Design review of the part built by this model. Coordinates are the model's own, in mm. A direction names the side the tool comes from. Coordinates: 2 decimals unless noted, no trailing zeros. Write each loop counter-clockwise with the first axis right and the second up, starting at its lowest first coordinate (ties: lowest second). Pieces come first, ordered by that corner, then holes. Notation, with made-up numbers: M -33,-36 L -25,-36 A34 cw -25,3 Z; hole C -31.5,-20.75 d11. An arc over 180 degrees is marked long. Write each question's results on one line, items separated by ' | '. Start each with the question number.
```python
from build123d import *

# Parameters (mm, degrees)
FILLET1_R       = 0.1
SKETCH3_W       = 0.74
SKETCH3_H       = 2.8
SKETCH4_W       = 0.74
SKETCH4_H       = 1.054964664
RECPAT_COUNT    = 2
RECPAT_ANGLE    = 90
THDSCHPAT_COUNT = 7
THDSCHPAT_PITCH = 0.5


with BuildPart() as part:
    # BodySke → Base-Revolve (revolve)
    with BuildSketch(Plane.XY):
        with BuildLine():
            Line((2.4, 1.5), (2.4, 2.8))
            Line((2.4, 2.8), (1.003501533, 2.8))
            ThreePointArc((1.003501533, 2.8), (0.873295971, 2.76653015), (0.775371599, 2.674418605))
            ThreePointArc((0.775371599, 2.674418605), (0.197753546, 1.392274756), (0, 0))
            Line((0, 0), (6.4, 0))
            Line((6.4, 0), (6.4, 1.5))
            Line((6.4, 1.5), (2.4, 1.5))
        make_face()
    revolve(axis=Axis((-25.4, 0, 0), (1, 0, 0)))

    # Fillet1
    fillet1_edges = [part.edges().sort_by_distance(p)[0] for p in [
        (2.4, -1.5, 0),
    ]]
    fillet(fillet1_edges, radius=FILLET1_R)

    # Sketch3 → Recess section 0
    with BuildSketch(Plane(origin=(0, 0, 0), x_dir=(0, 0, -1), z_dir=(1, 0, 0))):
        Rectangle(SKETCH3_W, SKETCH3_H)
    # Sketch4 → Recess section 1
    with BuildSketch(Plane(origin=(1.75, 0, 0), x_dir=(0, 0, -1), z_dir=(1, 0, 0))):
        Rectangle(SKETCH4_W, SKETCH4_H)
    recess = loft(mode=Mode.SUBTRACT)

    # RecPat: Recess ×2 about axis
    recpat_axis = Axis((0, 0, 0), (1, 0, 0))
    for i in range(1, RECPAT_COUNT):
        add(recess.rotate(recpat_axis, i * RECPAT_ANGLE / (RECPAT_COUNT - 1)), mode=Mode.SUBTRACT)

    # RecCorSke → RecessCore (revolve, cut)
    with BuildSketch(Plane.XY):
        Polygon((0, 0), (0, 0.678371921), (1.75, 0.556), (1.930655351, 0), align=None)
    revolve(axis=Axis((-3.175, 0, 0), (1, 0, 0)), mode=Mode.SUBTRACT)

    # ThdSchSke → ThreadSchematic (revolve, cut)
    with BuildSketch(Plane.XY):
        Polygon((3.4, -1.2195), (3.203591786, -1.5), (3.203591786, -1.875), (3.596408214, -1.875), (3.596408214, -1.5), align=None)
    threadschematic = revolve(axis=Axis((-3.175, 0, 0), (1, 0, 0)), mode=Mode.SUBTRACT)

    # ThdSchPat: ThreadSchematic ×7
    with Locations(*[(i * THDSCHPAT_PITCH, 0, 0) for i in range(1, THDSCHPAT_COUNT)]):
        add(threadschematic, mode=Mode.SUBTRACT)


solid = part.part
```
Item 1: For faces 1 (the conical face through (1.92, 0.03, 0.01)), 2 (the flat face through (2.4, 0, -2)), list the 3-axis set-ups (+Z, -Z, +X, -X, +Y, -Y) from which the entire face can be reached by the end or side of a thin tool; tool diameter is ignored.
Item 2: We need section A-A on z = 1.4. Count the separate pieces of the cut face and the enclosed holes in it, then the cut area to 3 significant figures.
Item 3: We need section B-B on x = 4.5. State the section outline as (y, z) points.
Item 4: Insertion check: pin 1 Ø1.5 at (x, y) = (5, -1) entering from -Z; pin 2 Ø3 at (y, z) = (-1.5, -1.5) entering from -X; pin 3 Ø3 at (x, z) = (3.5, 2) entering from +Y. Each pin has a flat end and moves straight along its axis. Give the tip position at first contact, or say it passes through.
Item 5: Wall thickness on L1, parallel to X at y = -0.7, z = -1.75; L2, parallel to Z at x = 0.5, y = -1.05; L3, parallel to Z at x = 0.75, y = -0.7: over which ranges is each line inside the solid? List them lowest first.
Answer:
1) face 1: -X | face 2: +X
2) separate pieces: 7 | enclosed holes: 0 | area: 11.8 mm^2
3) outline: C 0,0 d2.72
4) pin 1: stops at z = -1.48 | pin 2: stops at x = 0.05 | pin 3: stops at y = 2.62
5) L1: x = 0.37 to 2.4 | L2: z = -1.91 to -0.37, 0.37 to 1.91 | L3: z = -2.54 to -0.37, 0.37 to 2.54
